The listing builds one solid part. Answer for the finished solid, in the listing's coordinates (mm). A direction names the side the tool comes from. Give positions to 0.01 mm unless a question says otherwise; leave off trailing zeros. Write each loop counter-clockwise with the first axis right and the second up, starting at its lowest first coordinate (ties: lowest second). Pieces come first, ordered by that corner, then holes.
```python
from build123d import *

# Parameters (mm, degrees)
F0_W     = 56
F0_H     = 185
F1_DEPTH = 8
F2_SIZE  = 3
F4_D     = 6.5
F6_DEPTH = 25


with BuildPart() as f1:
    # F0 (on Front) → F1 (new body)
    with BuildSketch(Plane.XZ):
        Rectangle(F0_W, F0_H)
    extrude(amount=F1_DEPTH)

    # F2
    f2_edges = [f1.edges().sort_by_distance(p)[0] for p in [
        (28, -4, 92.5),
        (-28, -4, 92.5),
        (28, -4, -92.5),
        (-28, -4, -92.5),
    ]]
    chamfer(f2_edges, length=F2_SIZE)

    # F4 (through all)
    with Locations(Plane.XZ.offset(8)):
        with Locations((-17, -85.5), (23, -85.5), (23, -45.5), (-17, -45.5), (-17, 45.5), (23, 45.5), (23, 85.5), (-17, 85.5)):
            Hole(F4_D / 2)

    # F5 (on face) → F6 (cut)
    with BuildSketch(Plane.XZ.offset(8)):
        with BuildLine():
            ThreePointArc((6.5, 1), (3, -2.5), (6.5, -6))
            Line((6.5, -6), (6.5, 1))
        make_face()
        with BuildLine():
            Line((11.5, 1), (11.5, -6))
            ThreePointArc((11.5, -6), (13.9748737342, -4.9748737342), (15, -2.5))
            ThreePointArc((15, -2.5), (13.9748737342, -0.0251262658), (11.5, 1))
        make_face()
        with BuildLine():
            ThreePointArc((6.5, -29), (3, -32.5), (6.5, -36))
            Line((6.5, -36), (6.5, -29))
        make_face()
        with BuildLine():
            Line((11.5, -29), (11.5, -36))
            ThreePointArc((11.5, -36), (13.9748737342, -34.9748737342), (15, -32.5))
            ThreePointArc((15, -32.5), (13.9748737342, -30.0251262658), (11.5, -29))
        make_face()
        with BuildLine():
            Line((-17.81, -11.5), (-17.81, -18.5))
            ThreePointArc((-17.81, -18.5), (-15.3351262658, -17.4748737342), (-14.31, -15))
            ThreePointArc((-14.31, -15), (-15.3351262658, -12.5251262658), (-17.81, -11.5))
        make_face()
        with BuildLine():
            ThreePointArc((-22.81, 18.5), (-26.31, 15), (-22.81, 11.5))
            Line((-22.81, 11.5), (-22.81, 18.5))
        make_face()
        with BuildLine():
            Line((-17.81, 18.5), (-17.81, 11.5))
            ThreePointArc((-17.81, 11.5), (-15.3351262658, 12.5251262658), (-14.31, 15))
            ThreePointArc((-14.31, 15), (-15.3351262658, 17.4748737342), (-17.81, 18.5))
        make_face()
        with BuildLine():
            ThreePointArc((9, -4.9494897428), (7.8558735008, -5.7267021942), (6.5, -6))
            Line((6.5, -6), (11.5, -6))
            ThreePointArc((11.5, -6), (10.1441264992, -5.7267021942), (9, -4.9494897428))
        make_face()
        with BuildLine():
            Line((11.5, 1), (6.5, 1))
            ThreePointArc((6.5, 1), (7.8558735008, 0.7267021942), (9, -0.0505102572))
            ThreePointArc((9, -0.0505102572), (10.1441264992, 0.7267021942), (11.5, 1))
        make_face()
        with BuildLine():
            ThreePointArc((9, -34.9494897428), (7.8558735008, -35.7267021942), (6.5, -36))
            Line((6.5, -36), (11.5, -36))
            ThreePointArc((11.5, -36), (10.1441264992, -35.7267021942), (9, -34.9494897428))
        make_face()
        with BuildLine():
            Line((11.5, -29), (6.5, -29))
            ThreePointArc((6.5, -29), (7.8558735008, -29.2732978058), (9, -30.0505102572))
            ThreePointArc((9, -30.0505102572), (10.1441264992, -29.2732978058), (11.5, -29))
        make_face()
        with BuildLine():
            ThreePointArc((-20.31, -17.4494897428), (-21.4541264992, -18.2267021942), (-22.81, -18.5))
            Line((-22.81, -18.5), (-17.81, -18.5))
            ThreePointArc((-17.81, -18.5), (-19.1658735008, -18.2267021942), (-20.31, -17.4494897428))
        make_face()
        with BuildLine():
            Line((-17.81, -11.5), (-22.81, -11.5))
            ThreePointArc((-22.81, -11.5), (-21.4541264992, -11.7732978058), (-20.31, -12.5505102572))
            ThreePointArc((-20.31, -12.5505102572), (-19.1658735008, -11.7732978058), (-17.81, -11.5))
        make_face()
        with BuildLine():
            ThreePointArc((-20.31, 12.5505102572), (-21.4541264992, 11.7732978058), (-22.81, 11.5))
            Line((-22.81, 11.5), (-17.81, 11.5))
            ThreePointArc((-17.81, 11.5), (-19.1658735008, 11.7732978058), (-20.31, 12.5505102572))
        make_face()
        with BuildLine():
            Line((-17.81, 18.5), (-22.81, 18.5))
            ThreePointArc((-22.81, 18.5), (-21.4541264992, 18.2267021942), (-20.31, 17.4494897428))
            ThreePointArc((-20.31, 17.4494897428), (-19.1658735008, 18.2267021942), (-17.81, 18.5))
        make_face()
        with BuildLine():
            Line((6.5, 1), (6.5, -6))
            ThreePointArc((6.5, -6), (7.8558735008, -5.7267021942), (9, -4.9494897428))
            ThreePointArc((9, -4.9494897428), (8, -2.5), (9, -0.0505102572))
            ThreePointArc((9, -0.0505102572), (7.8558735008, 0.7267021942), (6.5, 1))
        make_face()
        with BuildLine():
            ThreePointArc((9, -4.9494897428), (10.1441264992, -5.7267021942), (11.5, -6))
            Line((11.5, -6), (11.5, 1))
            ThreePointArc((11.5, 1), (10.1441264992, 0.7267021942), (9, -0.0505102572))
            ThreePointArc((9, -0.0505102572), (9.7403703492, -1.1771243445), (10, -2.5))
            ThreePointArc((10, -2.5), (9.7403703492, -3.8228756555), (9, -4.9494897428))
        make_face()
        with BuildLine():
            Line((6.5, -29), (6.5, -36))
            ThreePointArc((6.5, -36), (7.8558735008, -35.7267021942), (9, -34.9494897428))
            ThreePointArc((9, -34.9494897428), (8, -32.5), (9, -30.0505102572))
            ThreePointArc((9, -30.0505102572), (7.8558735008, -29.2732978058), (6.5, -29))
        make_face()
        with BuildLine():
            ThreePointArc((9, -34.9494897428), (10.1441264992, -35.7267021942), (11.5, -36))
            Line((11.5, -36), (11.5, -29))
            ThreePointArc((11.5, -29), (10.1441264992, -29.2732978058), (9, -30.0505102572))
            ThreePointArc((9, -30.0505102572), (9.7403703492, -31.1771243445), (10, -32.5))
            ThreePointArc((10, -32.5), (9.7403703492, -33.8228756555), (9, -34.9494897428))
        make_face()
        with BuildLine():
            Line((-22.81, -11.5), (-22.81, -18.5))
            ThreePointArc((-22.81, -18.5), (-21.4541264992, -18.2267021942), (-20.31, -17.4494897428))
            ThreePointArc((-20.31, -17.4494897428), (-21.31, -15), (-20.31, -12.5505102572))
            ThreePointArc((-20.31, -12.5505102572), (-21.4541264992, -11.7732978058), (-22.81, -11.5))
        make_face()
        with BuildLine():
            ThreePointArc((-20.31, -17.4494897428), (-19.1658735008, -18.2267021942), (-17.81, -18.5))
            Line((-17.81, -18.5), (-17.81, -11.5))
            ThreePointArc((-17.81, -11.5), (-19.1658735008, -11.7732978058), (-20.31, -12.5505102572))
            ThreePointArc((-20.31, -12.5505102572), (-19.5696296508, -13.6771243445), (-19.31, -15))
            ThreePointArc((-19.31, -15), (-19.5696296508, -16.3228756555), (-20.31, -17.4494897428))
        make_face()
        with BuildLine():
            Line((-22.81, 18.5), (-22.81, 11.5))
            ThreePointArc((-22.81, 11.5), (-21.4541264992, 11.7732978058), (-20.31, 12.5505102572))
            ThreePointArc((-20.31, 12.5505102572), (-21.31, 15), (-20.31, 17.4494897428))
            ThreePointArc((-20.31, 17.4494897428), (-21.4541264992, 18.2267021942), (-22.81, 18.5))
        make_face()
        with BuildLine():
            ThreePointArc((-20.31, 12.5505102572), (-19.1658735008, 11.7732978058), (-17.81, 11.5))
            Line((-17.81, 11.5), (-17.81, 18.5))
            ThreePointArc((-17.81, 18.5), (-19.1658735008, 18.2267021942), (-20.31, 17.4494897428))
            ThreePointArc((-20.31, 17.4494897428), (-19.5696296508, 16.3228756555), (-19.31, 15))
            ThreePointArc((-19.31, 15), (-19.5696296508, 13.6771243445), (-20.31, 12.5505102572))
        make_face()
        with BuildLine():
            ThreePointArc((-22.81, -11.5), (-26.31, -15), (-22.81, -18.5))
            Line((-22.81, -18.5), (-22.81, -11.5))
        make_face()
        with BuildLine():
            ThreePointArc((-20.31, -12.5505102572), (-21.31, -15), (-20.31, -17.4494897428))
            ThreePointArc((-20.31, -17.4494897428), (-19.5696296508, -16.3228756555), (-19.31, -15))
            ThreePointArc((-19.31, -15), (-19.5696296508, -13.6771243445), (-20.31, -12.5505102572))
        make_face()
        with BuildLine():
            ThreePointArc((-20.31, 17.4494897428), (-21.31, 15), (-20.31, 12.5505102572))
            ThreePointArc((-20.31, 12.5505102572), (-19.5696296508, 13.6771243445), (-19.31, 15))
            ThreePointArc((-19.31, 15), (-19.5696296508, 16.3228756555), (-20.31, 17.4494897428))
        make_face()
        with BuildLine():
            ThreePointArc((9, -0.0505102572), (8, -2.5), (9, -4.9494897428))
            ThreePointArc((9, -4.9494897428), (9.7403703492, -3.8228756555), (10, -2.5))
            ThreePointArc((10, -2.5), (9.7403703492, -1.1771243445), (9, -0.0505102572))
        make_face()
        with BuildLine():
            ThreePointArc((9, -30.0505102572), (8, -32.5), (9, -34.9494897428))
            ThreePointArc((9, -34.9494897428), (9.7403703492, -33.8228756555), (10, -32.5))
            ThreePointArc((10, -32.5), (9.7403703492, -31.1771243445), (9, -30.0505102572))
        make_face()
    extrude(amount=-F6_DEPTH, mode=Mode.SUBTRACT)


solid = f1.part
```
Item 1: Determine the mould class of faces 3 (the face through (26.5, -3.9, -91)), 4 (the face through (-26.5, -3.9, 91)), 5 (the face through (3, -4.1, -32.4)) for opening direction X: pulls with the +X half, pulls with the -X half, needs draft (parallel to the pull), parting line crosses it, or undercut.
Conclusion:
face 3: pulls with the +X half
face 4: pulls with the -X half
face 5: undercut
Item 2: A cutting plane is placed at B-B, the plane y = -2. Count the separate pieces of the cut face and the enclosed holes in it, plus the area to 3 significant figures.
Conclusion:
separate pieces: 1
enclosed holes: 12
area: 9,780 mm2
Item 3: A cutting plane is placed at A-A, the plane z = 45.5. Give the vertices of the cut face in (x, y).
Conclusion:
outline: (-28, -8) - (-20.25, -8) - (-20.25, 0) - (-28, 0) - close; (-13.75, -8) - (19.75, -8) - (19.75, 0) - (-13.75, 0) - close; (26.25, -8) - (28, -8) - (28, 0) - (26.25, 0) - close
Item 4: Which of the six approach directions +Z, -Z, +X, -X, +Y, -Y give full straight-line access (tool end or side, diameter ignored) to faces 1 (the face through (9, -4, 1)), 2 (the face through (26.5, -3.9, 91))?
Conclusion:
face 1: +Y, -Y
face 2: +Z, +X, +Y, -Y
Item 5: Consider probe 1 along Z at (x, y) = (23, -1.5); probe 2 along Z at (x, y) = (6, -4.75); probe 3 along Z at (x, y) = (24, -3.25). Determine where each line is inside the solid, lowest interval first.
Conclusion:
probe 1: z = -92.5 to -88.75, -82.25 to -48.75, -42.25 to 42.25, 48.75 to 82.25, 88.75 to 92.5
probe 2: z = -92.5 to -35.96, -29.04 to -5.96, 0.96 to 92.5
probe 3: z = -92.5 to -88.59, -82.41 to -48.59, -42.41 to 42.41, 48.59 to 82.41, 88.59 to 92.5
Item 6: This flat-tipped pin is pushed along its axis until it touches: P1, Ø8.5, axis at x = -17, z = 45.5, coming from the +Y side. Where does it stop, or does it pass through?
Conclusion:
P1: stops at y = 0
